Geometry: see drawing. Coordinates: mm, zero at the bounding-box minimum. A direction names the side the tool comes from. Round coordinates to 2 decimals unless told otherwise and drop trailing zeros. Loops run counter-clockwise (first coordinate to the right, second up) from the corner with the lowest first, then second, coordinate; pieces in that order, holes last. Notation, with made-up numbers: (11.5, -1.5) - (36.5, -1.5) arc R8 ccw to (36.5, 11.5) - close; hole circle Ø3 at (4, 27). An arc over 180 degrees is marked (long way). Return JSON: item names as keys, results as strings. Group by question number.
1. Draft query along Z for the marked faces 4, 5 and 6. Return one class per face: +Z half, -Z half, draft (parallel to the pull), parting line (faces both ways), or undercut.
2. Section B-B on x = 41. Return loops of the section in (y, z), and give its area (4 significant figures).
3. Material intervals for probe 1 along Z at (x, y) = (30.5, 19); probe 2 along Z at (x, y) = (24, 51.5); probe 3 along Y at (x, z) = (32, 155.5), sorted ascending.
4. Section D-D on z = 115. Return loops of the section in (x, y), and give its area (3 significant figures).
5. First-contact query: pin 1 Ø5 at (x, y) = (15, 45.5) entering from +Z; pin 2 Ø20 at (x, y) = (19.5, 48.5) entering from -Z; pin 3 Ø22 at (x, z) = (14.5, 319.5) entering from +Y. Flat tips, straight axial feed; report the tip coordinate or a pass-through.
6. Section A-A on y = 25.5. Return loops of the section in (x, z).
7. Set-up query: the marked faces 1, 2 and 3. Return all of +Z, -Z, +X, -X, +Y, -Y with unobstructed straight access to the full face (end or side cutting, diameter ignored); none if empty.
8. Section C-C on y = 39. Return loops of the section in (x, z), and give its area (3 significant figures).
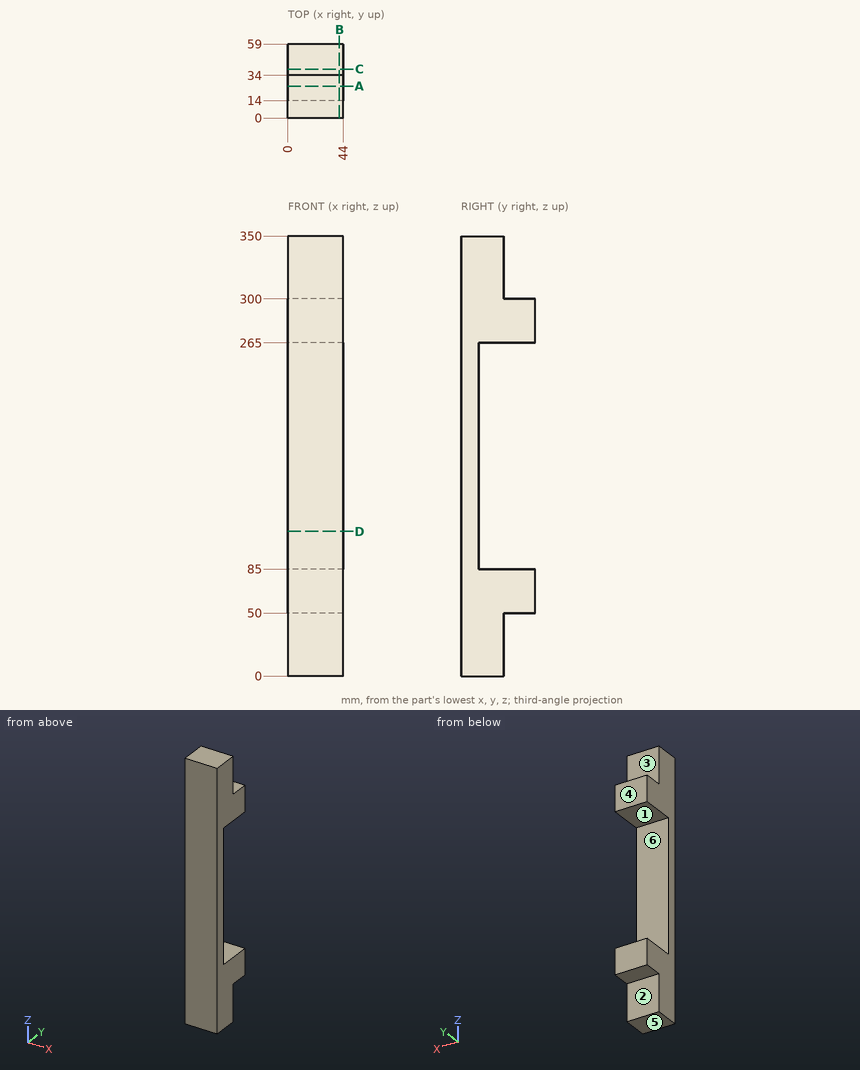
Taken from the geometry:
{
 "1": {"face 4": "draft", "face 5": "-Z half", "face 6": "undercut"},
 "2": {"outline": "(0, 0) - (34, 0) - (34, 50) - (59, 50) - (59, 85) - (14, 85) - (14, 265) - (59, 265) - (59, 300) - (34, 300) - (34, 350) - (0, 350) - close", "area": "10,050 mm2"},
 "3": {"probe 1": "0 to 85, 265 to 350", "probe 2": "50 to 85, 265 to 300", "probe 3": "0 to 14"},
 "4": {"outline": "(0, 0) - (44, 0) - (44, 14) - (0, 14) - close", "area": "616 mm2"},
 "5": {"pin 1": "z = 300", "pin 2": "z = 50", "pin 3": "y = 34"},
 "6": {"outline": "(0, 0) - (44, 0) - (44, 85) - (0, 85) - close; (0, 265) - (44, 265) - (44, 350) - (0, 350) - close"},
 "7": {"face 1": "+X, -X, +Y", "face 2": "-Z, +X, -X, +Y", "face 3": "+Z, +X, -X, +Y"},
 "8": {"outline": "(0, 50) - (44, 50) - (44, 85) - (0, 85) - close; (0, 265) - (44, 265) - (44, 300) - (0, 300) - close", "area": "3,080 mm2"}
}
